from build123d import *

# Parameters (mm, degrees)
SKETCH_1_R      = 2
EXTRUDE_1_DEPTH = 2
FILLET_1_R      = 1.5
FILLET_2_R      = 2.5


with BuildPart() as part:
    # 草图1 → 凸台-拉伸1 (new body)
    with BuildSketch(Plane.XY):
        with BuildLine():
            Line((7.071067812, 17.071067812), (10, 17.071067812))
            Line((10, 17.071067812), (10, 29))
            Line((10, 29), (-15, 29))
            Line((-15, 29), (-30, 29))
            Line((-30, 29), (-30, -29))
            Line((-30, -29), (-15, -29))
            Line((-15, -29), (10, -29))
            Line((10, -29), (10, 2.928932188))
            Line((10, 2.928932188), (7.071067812, 2.928932188))
            ThreePointArc((7.071067812, 2.928932188), (-10, 10), (7.071067812, 17.071067812))
        make_face()
        with Locations((5, -24)):
            Circle(SKETCH_1_R, mode=Mode.SUBTRACT)
        with Locations((-5, -24)):
            Circle(SKETCH_1_R, mode=Mode.SUBTRACT)
        with Locations((-5, 24)):
            Circle(SKETCH_1_R, mode=Mode.SUBTRACT)
        with Locations((5, 24)):
            Circle(SKETCH_1_R, mode=Mode.SUBTRACT)
        Polygon((-20, 24), (-17.5, 24), (-17.5, -24), (-22.5, -24), (-22.5, 24), align=None, mode=Mode.SUBTRACT)
    extrude(amount=EXTRUDE_1_DEPTH)

    # 圆角1
    fillet_1_edges = [part.edges().sort_by_distance(p)[0] for p in [
        (7.071067812, 2.928932188, 1),
        (10, 2.928932188, 1),
        (10, -29, 1),
        (-30, -29, 1),
        (-30, 29, 1),
        (10, 29, 1),
        (10, 17.071067812, 1),
        (7.071067812, 17.071067812, 1),
    ]]
    fillet(fillet_1_edges, radius=FILLET_1_R)

    # 圆角2
    fillet_2_edges = [part.edges().sort_by_distance(p)[0] for p in [
        (-17.5, -24, 1),
        (-22.5, -24, 1),
        (-22.5, 24, 1),
        (-17.5, 24, 1),
    ]]
    fillet(fillet_2_edges, radius=FILLET_2_R - 0.0001)  # a hair under: the kernel refuses the full size


solid = part.part
For this review, take the finished solid that the model builds, in its own axes (mm). A direction names the side the tool comes from. Round coordinates to 2 decimals unless told otherwise and drop trailing zeros. Loops run counter-clockwise (first coordinate to the right, second up) from the corner with the lowest first, then second, coordinate; pieces in that order, holes last. Notation, with made-up numbers: (50.5, 86) - (60.5, 86) arc R7 ccw to (60.5, 94) - close; hole circle Ø10 at (-14, 51). An arc over 180 degrees is marked (long way). One line per item, written item: value. Start each with the question number.
Item 1: Take a section at A-A (y = 10). Give the boundary of the cut face in (x, z).
Item 2: Take a section at C-C (x = 6). Give the boundary of the cut face in (y, z).
Item 3: Take a section at D-D (y = -25). Give the boundary of the cut face in (x, z).
Item 4: For L1, parallel to X at y = 10, z = 1.55; L2, parallel to Y at x = 4.5, z = 1.8; L3, parallel to Y at x = 0, z = 0.9, list the stretches that pass through material, from the lowest coordinate up.
Item 5: Take a section at B-B (z = 0.4). State how many separate pieces and enclosed holes the cut face has, plus the area to 3 significant figures.
Item 6: For faces 1 (the cylindrical face through (9.57, 28.55, 1.01)), 2 (the cylindrical face through (9.57, 2.48, 1.01)), 3 (the cylindrical face through (-22, 23, 1)), list the 3-axis set-ups (+Z, -Z, +X, -X, +Y, -Y) from which the entire face can be reached by the end or side of a thin tool; tool diameter is ignored.
Item 7: The part is to be moulded in two halves that separate along Y. For faces 4 (the flat face through (-22.5, 0, 1)), 5 (the cylindrical face through (-29.55, 28.57, 1.01)), 6 (the flat face through (-10, -29, 1)), say which applies: +Y half, -Y half, draft (parallel to the pull), parting line (faces both ways), or undercut.
Item 8: Clearance check with flat-ended pins moving along their axes: pin 1 Ø3 at (x, y) = (-5, -24) entering from +Z; pin 2 Ø6 at (x, y) = (2.5, 19.5) entering from +Z; pin 3 Ø1 at (y, z) = (6, 1) entering from +X. State where each tip first meets the part, or that it passes through.
Answer below:
1. outline: (-30, 0) - (-22.5, 0) - (-22.5, 2) - (-30, 2) - close; (-17.5, 0) - (-10, 0) - (-10, 2) - (-17.5, 2) - close
2. outline: (-29, 0) - (-25.73, 0) - (-25.73, 2) - (-29, 2) - close; (-22.27, 0) - (2, 0) - (2, 2) - (-22.27, 2) - close; (18, 0) - (22.27, 0) - (22.27, 2) - (18, 2) - close; (25.73, 0) - (29, 0) - (29, 2) - (25.73, 2) - close
3. outline: (-30, 0) - (-6.73, 0) - (-6.73, 2) - (-30, 2) - close; (-3.27, 0) - (3.27, 0) - (3.27, 2) - (-3.27, 2) - close; (6.73, 0) - (10, 0) - (10, 2) - (6.73, 2) - close
4. L1: x = -30 to -22.5, -17.5 to -10
4. L2: y = -29 to -25.94, -22.06 to 1.07, 18.93 to 22.06, 25.94 to 29
4. L3: y = -29 to 0, 20 to 29
5. separate pieces: 1
5. enclosed holes: 5
5. area: 1,710 mm2
6. face 1: +Z, -Z, +X, +Y
6. face 2: +Z, -Z, +X
6. face 3: +Z, -Z
7. face 4: undercut
7. face 5: +Y half
7. face 6: -Y half
8. pin 1: passes through
8. pin 2: stops at z = 2
8. pin 3: stops at x = -8.93
